from build123d import *

# Parameters (mm, degrees)
EXTRUDE_1_DEPTH     = 35
SKETCH_3_W          = 28
SKETCH_3_H          = 5
CUT_EXTRUDE_1_DEPTH = 119.559064219
SKETCH_4_R          = 2
CUT_EXTRUDE_2_DEPTH = 75.707768298


with BuildPart() as part:
    # 草图1 → 凸台-拉伸1 (new body)
    with BuildSketch(Plane.XY):
        with BuildLine():
            Line((-52.500003752, 27.500001563), (-52.500003752, 42.500001563))
            Line((-52.500003752, 42.500001563), (-47.500003752, 42.500001563))
            Line((-47.500003752, 42.500001563), (-47.500003752, 27.500001563))
            ThreePointArc((-47.500003752, 27.500001563), (-40.17767174, 9.822329823), (-22.5, 2.499998437))
            Line((-22.5, 2.499998437), (22.5, 2.499998437))
            ThreePointArc((22.5, 2.499998437), (40.17767174, 9.822329823), (47.500003752, 27.500001563))
            Line((47.500003752, 27.500001563), (47.500003752, 42.500001563))
            Line((47.500003752, 42.500001563), (52.500003752, 42.500001563))
            Line((52.500003752, 42.500001563), (52.500003752, 27.500001563))
            ThreePointArc((52.500003752, 27.500001563), (43.713203436, 6.286798128), (22.5, -2.499998437))
            Line((22.5, -2.499998437), (-22.5, -2.499998437))
            ThreePointArc((-22.5, -2.499998437), (-43.713203436, 6.286798128), (-52.500003752, 27.500001563))
        make_face()
    extrude(amount=EXTRUDE_1_DEPTH)

    # 草图3 → 切除-拉伸1 (cut, through all)
    with BuildSketch(Plane(origin=(52.500003752, 0, 0), x_dir=(0, 0, -1), z_dir=(1, 0, 0))):
        with Locations((-17.5, 36.000001563)):
            Rectangle(SKETCH_3_W, SKETCH_3_H)
    extrude(amount=-CUT_EXTRUDE_1_DEPTH, mode=Mode.SUBTRACT)

    # 草图4 → 切除-拉伸2 (cut, through all)
    with BuildSketch(Plane(origin=(0, 2.499998437, 0), x_dir=(1, 0, 0), z_dir=(0, 1, 0))):
        with Locations(Location((-10, -12.5, 0), (0, 0, 180))):
            Circle(SKETCH_4_R)
        with Locations(Location((-10, -22.5, 0), (0, 0, 180))):
            Circle(SKETCH_4_R)
        with Locations((10, -22.5)):
            Circle(SKETCH_4_R)
        with Locations((10, -12.5)):
            Circle(SKETCH_4_R)
    extrude(amount=-CUT_EXTRUDE_2_DEPTH, mode=Mode.SUBTRACT)


solid = part.part
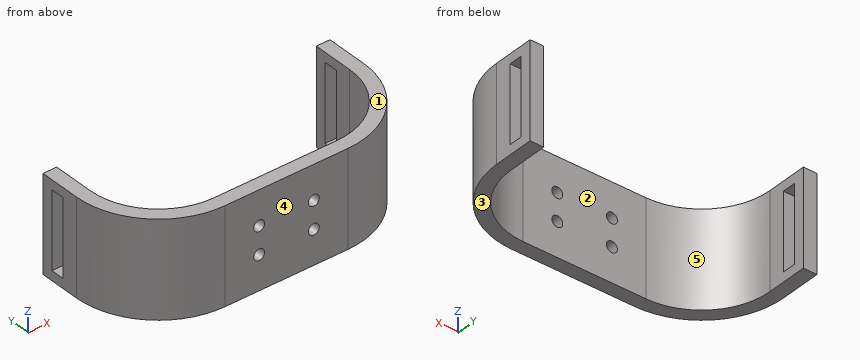
Build history of the part. All positions in model axes, mm. Face numbers are marked on the shaded views. A direction names the side the tool comes from. Give positions to 0.01 mm unless a question says otherwise; leave off trailing zeros. Order: outer loops, then holes, each group sorted by start corner. A loop starts at its lowest first (then second) coordinate and runs counter-clockwise, first axis right, second up. Notation, with made-up numbers: M -28.5,-22.75 L -2.5,-22.75 A16 cw -2.5,5.25 Z; hole C -23.75,50.25 d10. An arc over 180 degrees is marked long. Put each result on its own line as item: value.
Item 1: 3-axis set-ups, long thin cutter, end or side, ignore diameter. For the marked faces 4 and 5: which of +Z, -Z, +X, -X, +Y, -Y reach the whole face in a straight line?
From the geometry:
face 4: +Z, -Z, +X, -X, -Y
face 5: +Z, -Z, +Y
Item 2: Slice it at B-B, the plane x = -10. Write the cut outline in (y, z), plus the area to 3 significant figures.
From the geometry:
outline: M -2.5,0 L 2.5,0 L 2.5,10.5 L -2.5,10.5 Z; M -2.5,14.5 L 2.5,14.5 L 2.5,20.5 L -2.5,20.5 Z; M -2.5,24.5 L 2.5,24.5 L 2.5,35 L -2.5,35 Z
area: 135 mm2
Item 3: Slice it at A-A, the plane z = 12.5. Write the cut outline in (x, y).
From the geometry:
outline: M -52.5,27.5 A30 ccw -22.5,-2.5 L -12,-2.5 L -12,2.5 L -22.5,2.5 A25 cw -47.5,27.5 L -47.5,33.5 L -52.5,33.5 Z; M -52.5,38.5 L -47.5,38.5 L -47.5,42.5 L -52.5,42.5 Z; M -8,-2.5 L 8,-2.5 L 8,2.5 L -8,2.5 Z; M 12,-2.5 L 22.5,-2.5 A30 ccw 52.5,27.5 L 52.5,33.5 L 47.5,33.5 L 47.5,27.5 A25 cw 22.5,2.5 L 12,2.5 Z; M 47.5,38.5 L 52.5,38.5 L 52.5,42.5 L 47.5,42.5 Z
Item 4: Slice it at D-D, the plane y = 1. Write the cut outline in (x, z), plus the area to 3 significant figures.
From the geometry:
outline: M -36.56,0 L 36.56,0 L 36.56,35 L -36.56,35 Z; hole C -10,12.5 d4; hole C -10,22.5 d4; hole C 10,12.5 d4; hole C 10,22.5 d4
area: 2,510 mm2
Item 5: Two-plate mould, pull along Z, no slides. Class the marked faces 1, 2 and 3: +Z half, -Z half, draft (parallel to the pull), parting line (faces both ways), or undercut.
From the geometry:
face 1: +Z half
face 2: draft
face 3: -Z half
Item 6: Probe line 1 (Z direction, x = 10, y = -1); line 2 (X direction, y = 40, z = 11); line 3 (Y direction, x = 9, z = 26). List the from-to ranges inside material, lowest first. Write a range as [from, to].
From the geometry:
line 1: z = [0, 10.5], [14.5, 20.5], [24.5, 35]
line 2: x = [-52.5, -47.5], [47.5, 52.5]
line 3: y = [-2.5, 2.5]
Item 7: Flat gauge pins, fed straight in: pin 1 Ø4 at (x, z) = (51, 24) entering from -Y; pin 2 Ø4.5 at (x, z) = (-10, 22.5) entering from +Y; pin 3 Ø4 at (x, z) = (-50, 21.5) entering from -Y. Where does each tip first touch, or does it go through?
From the geometry:
pin 1: stops at y = 13.44
pin 2: stops at y = 2.5
pin 3: stops at y = 11.7
Item 8: Slice it at C-C, the plane y = 13.5. Write the cut outline in (x, z), plus the area to 3 significant figures.
From the geometry:
outline: M -49.03,0 L -43.21,0 L -43.21,35 L -49.03,35 Z; M 43.21,0 L 49.03,0 L 49.03,35 L 43.21,35 Z
area: 407 mm2
